from build123d import *

# Parameters (mm, degrees)
SKETCH_1_W          = 30
SKETCH_1_H          = 3
EXTRUDE_2_DEPTH     = 11
SKETCH_1_5_W        = 30
SKETCH_1_5_H        = 10
EXTRUDE_3_DEPTH     = 3
EXTRUDE_4_DEPTH     = 30
CUT_EXTRUDE_1_DEPTH = 15


with BuildPart() as part:
    # 草图1 → 凸台-拉伸2 (new body)
    with BuildSketch(Plane(origin=(0, 0, 0), x_dir=(1, 0, 0), z_dir=(0, 1, 0))):
        with Locations((15, -11.5)):
            Rectangle(SKETCH_1_W, SKETCH_1_H)
    extrude(amount=-EXTRUDE_2_DEPTH)

    # 草图1<5> → 凸台-拉伸3 (add)
    with BuildSketch(Plane(origin=(0, 0, 0), x_dir=(1, 0, 0), z_dir=(0, 1, 0))):
        with Locations((15, -5)):
            Rectangle(SKETCH_1_5_W, SKETCH_1_5_H)
    extrude(amount=-EXTRUDE_3_DEPTH)

    # 草图3 → 凸台-拉伸4 (add)
    with BuildSketch(Plane.ZY):
        Polygon((0, 0), (0, 99), (40, 99), (40, 96), (13, 96), (13, 0), align=None)
    extrude(amount=-EXTRUDE_4_DEPTH)

    # 草图3<4> → 切除-拉伸1 (cut)
    with BuildSketch(Plane.ZY):
        Polygon((0, 0), (0, 99), (40, 99), (40, 96), (13, 96), (13, 0), align=None)
    extrude(amount=-CUT_EXTRUDE_1_DEPTH, mode=Mode.SUBTRACT)


solid = part.part
Work out the finished part from the listing and answer in its coordinate system (mm). A direction names the side the tool comes from. Round coordinates to 2 decimals unless told otherwise and drop trailing zeros. Write each loop counter-clockwise with the first axis right and the second up, starting at its lowest first coordinate (ties: lowest second). Pieces come first, ordered by that corner, then holes. Notation, with made-up numbers: (72, -16) - (91, -16) arc R16 cw to (91, -8) - close; hole circle Ø8 at (2, 20). An arc over 180 degrees is marked (long way). Answer in a Markdown table with one row per item. Add a question column.
1. A cutting plane is placed at A-A, the plane x = 19. Determine the outline of the cut face in (y, z), and give its area (3 significant figures).
2. Find the intervals of material crossed by line 1 along Y through (x, z) = (17.5, 27); line 2 along Z through (x, y) = (19.5, 14); line 3 along X through (y, z) = (33.5, 12), in increasing order. Write a range as from..to.
3. A cutting plane is placed at D-D, the plane x = 13. Determine the outline of the cut face in (y, z).
4. Given pin 1 (2 mm diameter, centred on x = 11, z = 9, fed in from +Y); pin 2 (9 mm diameter, centred on x = 18, y = 29.5, fed in from +Z); pin 3 (4 mm diameter, centred on x = 25.5, z = 19.5, fed in from -Y), each flat-ended and moving along its own axis, determine where each tip first touches the part or whether it passes through.
5. A cutting plane is placed at B-B, the plane z = 6.5. Determine the outline of the cut face in (x, y), and give its area (4 significant figures).
6. A cutting plane is placed at C-C, the plane y = 14.5. Determine the outline of the cut face in (x, z), and give its area (3 significant figures).
7. For faces 1 (the flat face through (21, 43, 13)), 2 (the flat face through (15, 53, 8)), 3 (the flat face through (15, -7, 10)), determine the directions among +Z, -Z, +X, -X, +Y, -Y from which every point of the face is accessible in a straight line to the end or side of a thin tool.
Worked out:
| question | item | result |
|---|---|---|
| 1 | outline | (-11, 10) - (-3, 10) - (-3, 0) - (99, 0) - (99, 40) - (96, 40) - (96, 13) - (-11, 13) - close |
| 1 | area | 1,430 mm^2 |
| 2 | line 1 | 96..99 |
| 2 | line 2 | 0..13 |
| 2 | line 3 | 15..30 |
| 3 | outline | (-11, 10) - (-3, 10) - (-3, 0) - (0, 0) - (0, 13) - (-11, 13) - close |
| 4 | pin 1 | y = 0 |
| 4 | pin 2 | z = 13 |
| 4 | pin 3 | y = 96 |
| 5 | outline | (0, -3) - (30, -3) - (30, 99) - (15, 99) - (15, 0) - (0, 0) - close |
| 5 | area | 1,575 mm^2 |
| 6 | outline | (15, 0) - (30, 0) - (30, 13) - (15, 13) - close |
| 6 | area | 195 mm^2 |
| 7 | face 1 | +Z, +X, -X, -Y |
| 7 | face 2 | +Z, -Z, -X, +Y |
| 7 | face 3 | -Z, +X, -X, -Y |
